from build123d import *

# Parameters (mm, degrees)
F1_DEPTH = 133.35
F2_R     = 4.5466
F3_DEPTH = 25.4
F4_R     = 4.5466
F5_DEPTH = 25.4
F6_R     = 2.54
F7_R     = 3.175


with BuildPart() as f1:
    # F0 (on Front) → F1 (new body)
    with BuildSketch(Plane.XZ):
        Polygon((-29.6893073604, 12.910717619), (-29.6893073604, -25.189282381), (-23.3393073604, -25.189282381), (-23.3393073604, 6.560717619), (14.7606926396, 6.560717619), (14.7606926396, 12.910717619), align=None)
    extrude(amount=F1_DEPTH)

    # F2 (on face) → F3 (cut)
    with BuildSketch(Plane(origin=(-29.6893073604, 0, 0), x_dir=(0, -1, 0), z_dir=(-1, 0, 0))):
        with Locations((25.4, -14.076782381)):
            Circle(F2_R)
        with Locations((88.9, -14.076782381)):
            Circle(F2_R)
    extrude(amount=-F3_DEPTH, mode=Mode.SUBTRACT)

    # F4 (on face) → F5 (cut)
    with BuildSketch(Plane.XY.offset(12.910717619)):
        with Locations((2.0606926396, -120.65)):
            Circle(F4_R)
        with Locations((2.0606926396, -19.05)):
            Circle(F4_R)
    extrude(amount=-F5_DEPTH, mode=Mode.SUBTRACT)

    # F6
    f6_edges = [f1.edges().sort_by_distance(p)[0] for p in [
        (14.760693, -133.35, 9.735718),
        (-7.464307, -133.35, 12.910718),
        (-7.464307, 0, 12.910718),
        (14.760693, 0, 9.735718),
    ]]
    fillet(f6_edges, radius=F6_R)

    # F7
    f7_edges = [f1.edges().sort_by_distance(p)[0] for p in [
        (-26.514307, -133.35, -25.189282),
        (-26.514307, 0, -25.189282),
        (-23.339307, -66.675, 6.560718),
    ]]
    fillet(f7_edges, radius=F7_R)


solid = f1.part
Read the model definition and answer for the solid it produces. Units are mm, in the model's axes. A direction names the side the tool comes from. Give positions to 0.01 mm unless a question says otherwise; leave off trailing zeros. Write each loop counter-clockwise with the first axis right and the second up, starting at its lowest first coordinate (ties: lowest second). Pieces come first, ordered by that corner, then holes. Notation, with made-up numbers: M 5.5,58.25 L 37.5,58.25 A6 cw 37.5,62.25 Z; hole C -20.75,15 d9. An arc over 180 degrees is marked long. One line per item, written item: value. Start each with the question number.
(1) Find section A-A (y = -88.9). Determine the outline of the cut face in (x, z) (3 decimals), plus the area to 3 significant figures.
(2) Determine the mould class of faces 1 (the flat face through (-24, 0, 0)), 2 (the cylindrical face through (-26.47, -0.905, -24.235)), 3 (the cylindrical face through (-26.559, -20.858, -13.877)) for opening direction Z: pulls with the +Z half, pulls with the -Z half, needs draft (parallel to the pull), parting line crosses it, or undercut.
(3) Find section C-C (z = -3). Determine the outline of the cut face in (x, y).
(4) Find section D-D (x = -25). Determine the outline of the cut face in (y, z) (3 decimals).
(5) Find the intervals of material crossed by line 1 (Y direction, x = 2, z = 8.5); line 2 (Z direction, x = -26, y = -25.4); line 3 (Z direction, x = -8.5, y = -119), in increasing order.
(6) A tool of negligible diameter and unlimited length cuts with its end or side. For faces 4 (the flat face through (-3, -66, 6.561)), 5 (the flat face through (-29.689, -66, -6)), from which of +Z, -Z, +X, -X, +Y, -Y can it reach the whole face along a straight path? Write none if from no direction.
(7) Flat-ended cylindrical pins translate along their axes: pin 1 Ø7.5 at (x, y) = (2.06, -120.65) entering from +Z; pin 2 Ø12 at (x, y) = (2.06, -19.05) entering from +Z; pin 3 Ø12 at (y, z) = (-88.9, -14.08) entering from +X; pin 4 Ø4 at (y, z) = (-89.5, 3) entering from +X. Find the tip coordinate at first contact, or state that the pin passes through.
(8) Find section B-B (x = 2). Determine the outline of the cut face in (y, z), plus the area to 3 significant figures.
Results below:
1. outline: M -29.689,-25.189 L -23.339,-25.189 L -23.339,-18.623 L -29.689,-18.623 Z; M -29.689,-9.53 L -23.339,-9.53 L -23.339,3.386 A3.175 cw -20.164,6.561 L 14.761,6.561 L 14.761,12.911 L -29.689,12.911 Z
1. area: 428 mm^2
2. face 1: needs draft
2. face 2: pulls with the -Z half
2. face 3: undercut
3. outline: M -29.69,-133.35 L -23.34,-133.35 L -23.34,0 L -29.69,0 Z
4. outline: M -133.35,-22.014 A3.175 ccw -130.175,-25.189 L -3.175,-25.189 A3.175 ccw 0,-22.014 L 0,10.371 A2.54 ccw -2.54,12.911 L -130.81,12.911 A2.54 ccw -133.35,10.371 Z; hole C -88.9,-14.077 d9.093; hole C -25.4,-14.077 d9.093
5. line 1: y = -133.35 to -125.2, -116.1 to -23.6, -14.5 to 0
5. line 2: z = -25.19 to -18.62, -9.53 to 12.91
5. line 3: z = 6.56 to 12.91
6. face 4: -Z, +X, +Y, -Y
6. face 5: +Z, -Z, -X, +Y, -Y
7. pin 1: passes through
7. pin 2: stops at z = 12.91
7. pin 3: stops at x = -23.34
7. pin 4: stops at x = -22.9
8. outline: M -133.35,6.56 L -125.2,6.56 L -125.2,12.91 L -130.81,12.91 A2.54 ccw -133.35,10.37 Z; M -116.1,6.56 L -23.6,6.56 L -23.6,12.91 L -116.1,12.91 Z; M -14.5,6.56 L 0,6.56 L 0,10.37 A2.54 ccw -2.54,12.91 L -14.5,12.91 Z
8. area: 729 mm^2
